Autodesk Inventor part; units mm, degrees
ref_plane "YZ Plane" through (0, 0, 0) normal (1, 0, 0) x (0, 1, 0)
ref_plane "XZ Plane" through (0, 0, 0) normal (0, 1, 0) x (-1, 0, 0)
ref_plane "XY Plane" through (0, 0, 0) normal (0, 0, 1) x (1, 0, 0)
sketch "Sketch1" plane through (0, 0, 0) normal (0, 1, 0) x (-1, 0, 0)
  line L0 (18.4, 24.2) -> (-18.4, 24.2)
  line L1 (-18.4, 24.2) -> (-18.4, -24.2)
  line L2 (-18.4, -24.2) -> (18.4, -24.2)
  line L3 (18.4, -24.2) -> (18.4, 24.2)
  point P0 (0, 0)
  point P1 (-18.4, 0)
  point P2 (0, -24.2)
  dimension "d0" = 48.4
  dimension "d1" = 36.8
extrude "Extrusion1" add sketch "Sketch1" along normal blind 3
sketch "Sketch2" plane through (0, 3, 0) normal (0, 1, 0) x (1, 0, 0)
  line L0 (-18.4, -24.2) -> (18.4, -24.2)
  line L1 (-18.4, 24.2) -> (-18.4, -24.2)
  line L2 (18.4, 24.2) -> (-18.4, 24.2)
  line L3 (18.4, -24.2) -> (18.4, 24.2)
  point P0 (0, 0)
  point P1 (-12.4, -20.2)
  point P2 (-12.4, 20.2)
  point P3 (12.4, -20.2)
  point P4 (12.4, 20.2)
  dimension "d4" = 4
  dimension "d5" = 6
  dimension "d6" = 6
  dimension "d7" = 4
  dimension "d8" = 6
  dimension "d9" = 4
  dimension "d10" = 6
  dimension "d11" = 4
hole "Hole1" at (-12.4, 3, 20.2) at (-12.4, 3, -20.2) at (12.4, 3, 20.2) at (12.4, 3, -20.2) direction (0, -1, 0) diameter 2 end through all
sketch "Sketch3" plane through (0, 3, 0) normal (0, 1, 0) x (1, 0, 0)
  line L0 (-18.4, 24.2) -> (-18.4, -24.2)
  line L1 (-18.4, -24.2) -> (18.4, -24.2)
  line L2 (18.4, 24.2) -> (-18.4, 24.2)
  circle A0 centre (-4.4, 0) radius 7.5
  circle A1 centre (-4.4, 0) radius 12.5
  point P0 (0, 0)
  dimension "d19" = 14
  dimension "d20" = 24.2
  dimension "d21" = 24.2
  dimension "d22" = 15
  dimension "d23" = 25
extrude "Extrusion2" add sketch "Sketch3" along normal blind 25
sketch "Sketch4" plane through (-4.4, 3, 0) normal (0, 1, 0) x (1, 0, 0)
  circle A0 centre (0, 0) radius 7.5
  point P0 (4.4, 0)
extrude "Extrusion3" cut sketch "Sketch4" against normal blind 35
sketch "Sketch5" plane through (-4.4, 28, 0) normal (0, 1, 0) x (1, 0, 0)
  circle A0 centre (0, 0) radius 10
  point P0 (4.4, 0)
  dimension "d29" = 20
extrude "Extrusion4" cut sketch "Sketch5" against normal blind 4
sketch "Sketch8" plane through (0, 0, 0) normal (0, -1, 0) x (1, 0, 0)
  circle A0 centre (-4.4, 0) radius 7.5
  circle A1 centre (-4.4, 0) radius 10
  point P0 (0, 0)
  dimension "d32" = 20
extrude "Extrusion5" cut sketch "Sketch8" against normal blind 4
fillet "Fillet2" radius 8 1 edges at (-16.9, 3, 0)
properties part number "Tube"
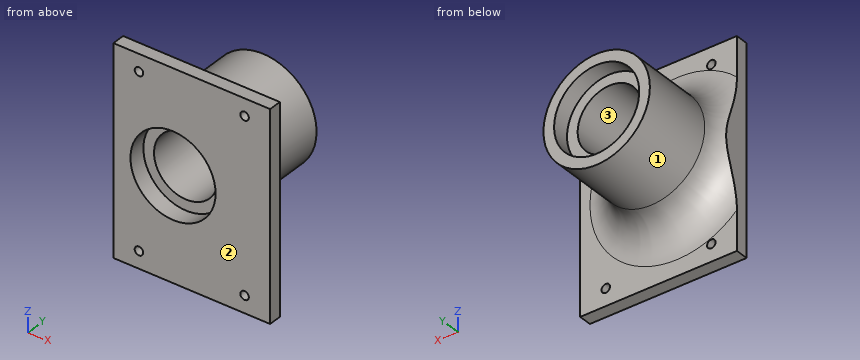
Geometry check sheet. Reference: the model listing, model coordinates, mm. Face numbers are marked on the shaded views. Round coordinates to 2 decimals unless told otherwise and drop trailing zeros. Order: outer loops, then holes, each group sorted by start corner. A loop starts at its lowest first (then second) coordinate and runs counter-clockwise, first axis right, second up. Notation, with made-up numbers: M -1.75,28.25 L 36.25,28.25 A21 cw 36.25,47.25 Z; hole C 57,67 d3. An arc over 180 degrees is marked long. Write each question's results on one line, items separated by ' | '. Start each with the question number.
1. Draft check along Z on the marked faces 1, 2 and 3. Enter one of: pulls with the +Z half, pulls with the -Z half, needs draft (parallel to the pull), parting line crosses it, or undercut.
2. Material ranges on L1, parallel to X at y = 1.8, z = -20.2; L2, parallel to X at y = 26.45, z = 0; L3, parallel to X at y = 27, z = -2.5, recorded low to high. Write a range as from..to.
3. Cross-section at B-B on x = -4.4. Record the boundary of the cut face in (y, z), plus the area to 3 significant figures.
4. Cross-section at A-A on z = 0. Record the boundary of the cut face in (x, y), plus the area to 3 significant figures.
5. Cross-section at D-D on x = 12.4. Give the number of separate pieces and of enclosed holes in the cut face, plus the area to 3 significant figures.
6. Go/stop test with flat-tipped pins: P1, Ø2.5, axis at x = 12.4, z = -20.2, coming from the -Y side; P2, Ø5, axis at y = 20, z = -11, coming from the -X side; P3, Ø4, axis at x = 12.5, z = -8.5, coming from the +Y side; P4, Ø12, axis at x = -12.5, y = 14.5, coming from the -Z side. Record where each tip stops, or that it passes through.
7. Cross-section at C-C on y = 25. Record the boundary of the cut face in (x, z), plus the area to 3 significant figures.
Resolved:
1) face 1: parting line crosses it | face 2: needs draft | face 3: undercut
2) L1: -18.4..-13.4, -11.4..11.4, 13.4..18.4 | L2: -16.9..-14.4, 5.6..8.1 | L3: -16.65..-14.08, 5.28..7.85
3) outline: M 0,-24.2 L 3,-24.2 L 3,-20.5 A8 cw 11,-12.5 L 28,-12.5 L 28,-10 L 24,-10 L 24,-7.5 L 4,-7.5 L 4,-10 L 0,-10 Z; M 0,10 L 4,10 L 4,7.5 L 24,7.5 L 24,10 L 28,10 L 28,12.5 L 11,12.5 A8 cw 3,20.5 L 3,24.2 L 0,24.2 Z | area: 338 mm2
4) outline: M -18.4,0 L -14.4,0 L -14.4,4 L -11.9,4 L -11.9,24 L -14.4,24 L -14.4,28 L -16.9,28 L -16.9,11 A8 cw -18.4,6.34 Z; M 3.1,4 L 5.6,4 L 5.6,0 L 18.4,0 L 18.4,3 L 16.1,3 A8 cw 8.1,11 L 8.1,28 L 5.6,28 L 5.6,24 L 3.1,24 Z | area: 296 mm2
5) separate pieces: 3 | enclosed holes: 0 | area: 144 mm2
6) P1: y = 0 | P2: x = -13.57 | P3: y = 3.85 | P4: z = -12.32
7) outline: C -4.4,0 d25; hole C -4.4,0 d20 | area: 177 mm2
